from build123d import *

# Parameters (mm, degrees)
F0_W     = 0.6
F0_H     = 1.8
F1_DEPTH = 6.5
F0_R     = 10
F0_R_2   = 8
F2_DEPTH = 5


with BuildPart() as f1:
    # F0 (on Top) → F1 (new body)
    with BuildSketch(Plane.XY):
        with Locations((-9, 0)):
            Rectangle(F0_W, F0_H)
    extrude(amount=F1_DEPTH)



with BuildPart() as f1b:
    # F0 (on Top) → F1, piece 2 (new body)
    with BuildSketch(Plane.XY):
        with Locations((9, 0)):
            Rectangle(F0_W, F0_H)
    extrude(amount=F1_DEPTH)


with BuildPart() as f1_1:
    add(f1.part)

    add(f1b.part)  # F2 merges F1b
    # F0 (on Top) → F2 (join)
    with BuildSketch(Plane.XY):
        Circle(F0_R)
        with Locations((-9, 0)):
            Rectangle(F0_W, F0_H, mode=Mode.SUBTRACT)
        Circle(F0_R_2, mode=Mode.SUBTRACT)
        with Locations((9, 0)):
            Rectangle(F0_W, F0_H, mode=Mode.SUBTRACT)
    extrude(amount=F2_DEPTH)


solid = f1_1.part
Build history of the part. All positions in model axes, mm. A direction names the side the tool comes from. Give positions to 0.01 mm unless a question says otherwise; leave off trailing zeros. Loops run counter-clockwise (first coordinate to the right, second up) from the corner with the lowest first, then second, coordinate; pieces in that order, holes last. Notation, with made-up numbers: (36.5, -5) -> (65.5, -5) arc R25 ccw to (65.5, 14) -> close; hole circle Ø2 at (-7.5, -0.75). An arc over 180 degrees is marked (long way). Answer in a Markdown table with one row per item.
Item 1: Flat gauge pins, fed straight in: P1, Ø1.5, axis at y = -6.5, z = 4.5, coming from the +X side; P2, Ø0.5, axis at x = -9, z = 5.5, coming from the +Y side; P3, Ø1.2, axis at y = 0, z = 6, coming from the -X side. Where does each tip first touch, or does it go through?
Findings below:
| item | result |
|---|---|
| P1 | stops at x = 8.18 |
| P2 | stops at y = 0.9 |
| P3 | stops at x = -9.3 |
Item 2: Slice it at A-A on x = 0. Write the cut outline in (y, z), plus the area to 3 significant figures.
Findings below:
| item | result |
|---|---|
| outline | (-10, 0) -> (-8, 0) -> (-8, 5) -> (-10, 5) -> close; (8, 0) -> (10, 0) -> (10, 5) -> (8, 5) -> close |
| area | 20.0 mm² |
Item 3: Slice it at B-B on y = 0. Write the cut outline in (x, z), plus the area to 3 significant figures.
Findings below:
| item | result |
|---|---|
| outline | (-10, 0) -> (-8, 0) -> (-8, 5) -> (-8.7, 5) -> (-8.7, 6.5) -> (-9.3, 6.5) -> (-9.3, 5) -> (-10, 5) -> close; (8, 0) -> (10, 0) -> (10, 5) -> (9.3, 5) -> (9.3, 6.5) -> (8.7, 6.5) -> (8.7, 5) -> (8, 5) -> close |
| area | 21.8 mm² |
Item 4: Slice it at D-D on x = 6.25. Write the cut outline in (y, z), plus the area to 3 significant figures.
Findings below:
| item | result |
|---|---|
| outline | (-7.81, 0) -> (-4.99, 0) -> (-4.99, 5) -> (-7.81, 5) -> close; (4.99, 0) -> (7.81, 0) -> (7.81, 5) -> (4.99, 5) -> close |
| area | 28.1 mm² |
Item 5: Slice it at C-C on z = 2.5. Write the cut outline in (x, y), plus the area to 3 significant figures.
Findings below:
| item | result |
|---|---|
| outline | circle Ø20 at (0, 0); hole circle Ø16 at (0, 0) |
| area | 113 mm² |
Item 6: Tool access for faces 5 (the cylindrical face through (-2.17, -9.76, 2.46)), 6 (the flat face through (8.7, 0, 6)), 7 (the flat face through (-9.3, 0, 6)): list every direction of +Z, -Z, +X, -X, +Y, -Y with a clear straight run to the whole face (end or side of a thin tool).
Findings below:
| item | result |
|---|---|
| face 5 | +Z, -Z |
| face 6 | +Z, +Y, -Y |
| face 7 | +Z, -X, +Y, -Y |
Item 7: Probe line 1 along Y through (x, z) = (0, 2.3); line 2 along X through (y, z) = (-1.75, 4.75); line 3 along Z through (x, y) = (-3.5, 8.5). List the from-to ranges inside material, lowest first. Write a range as [from, to].
Findings below:
| item | result |
|---|---|
| line 1 | y = [-10, -8], [8, 10] |
| line 2 | x = [-9.85, -7.81], [7.81, 9.85] |
| line 3 | z = [0, 5] |
Item 8: Mould opens along X. For faces 1 (the flat face through (-8.7, 0, 6)), 2 (the cylindrical face through (-1.73, -7.81, 2.46)), 3 (the flat face through (0, 8.2, 0)), 4 (the flat face through (9.3, 0, 6)) say: pulls with the +X half, pulls with the -X half, needs draft (parallel to the pull), parting line crosses it, or undercut.
Findings below:
| item | result |
|---|---|
| face 1 | undercut |
| face 2 | undercut |
| face 3 | needs draft |
| face 4 | pulls with the +X half |
